from build123d import *

# Parameters (mm, degrees)
SKETCH2_W                                           = 150
SKETCH2_H                                           = 30
BOSS_EXTRUDE1_DEPTH                                 = 20
SKETCH3_R                                           = 13.75
CUT_EXTRUDE1_DEPTH                                  = 13
LPATTERN1_COUNT                                     = 5
LPATTERN1_PITCH                                     = 30
CBORE_FOR_M4_HEX_SOCKET_HEAD_CAP_SCREW1_D           = 4.5
CBORE_FOR_M4_HEX_SOCKET_HEAD_CAP_SCREW1_CBORE_D     = 8
CBORE_FOR_M4_HEX_SOCKET_HEAD_CAP_SCREW1_CBORE_DEPTH = 4.4
LPATTERN2_COUNT                                     = 2
LPATTERN2_PITCH                                     = 120
SKETCH7_W                                           = 181.12901383
SKETCH7_H                                           = 4
CUT_EXTRUDE3_DEPTH                                  = 13
SKETCH8_W                                           = 4
SKETCH8_H                                           = 50
CUT_EXTRUDE4_DEPTH                                  = 13
LPATTERN3_COUNT                                     = 5
LPATTERN3_PITCH                                     = 30


with BuildPart() as part:
    # Sketch2 → Boss-Extrude1 (new body)
    with BuildSketch(Plane(origin=(0, 0, 0), x_dir=(1, 0, 0), z_dir=(0, 1, 0))):
        Rectangle(SKETCH2_W, SKETCH2_H)
    extrude(amount=BOSS_EXTRUDE1_DEPTH)

    # Sketch3 → Cut-Extrude1 (cut)
    with BuildSketch(Plane(origin=(0, 20, 0), x_dir=(1, 0, 0), z_dir=(0, 1, 0))):
        with Locations(Location((-60, 0, 0), (0, 0, 270))):
            Circle(SKETCH3_R)
    cut_extrude1 = extrude(amount=-CUT_EXTRUDE1_DEPTH, mode=Mode.SUBTRACT)

    # LPattern1: Cut-Extrude1 ×5
    with Locations(*[(i * LPATTERN1_PITCH, 0, 0) for i in range(1, LPATTERN1_COUNT)]):
        add(cut_extrude1, mode=Mode.SUBTRACT)

    # CBORE for M4 Hex Socket Head Cap Screw1 (through all)
    with Locations(Plane(origin=(0, 7, 0), x_dir=(-1, 0, 0), z_dir=(0, 1, 0))):
        with Locations((60, 0)):
            cbore_for_m4_hex_socket_head_cap_screw1 = CounterBoreHole(CBORE_FOR_M4_HEX_SOCKET_HEAD_CAP_SCREW1_D / 2, CBORE_FOR_M4_HEX_SOCKET_HEAD_CAP_SCREW1_CBORE_D / 2, CBORE_FOR_M4_HEX_SOCKET_HEAD_CAP_SCREW1_CBORE_DEPTH)

    # LPattern2: CBORE for M4 Hex Socket Head Cap Screw1 ×2
    with Locations(*[(i * LPATTERN2_PITCH, 0, 0) for i in range(1, LPATTERN2_COUNT)]):
        add(cbore_for_m4_hex_socket_head_cap_screw1, mode=Mode.SUBTRACT)

    # Sketch7 → Cut-Extrude3 (cut)
    with BuildSketch(Plane(origin=(0, 20, 0), x_dir=(1, 0, 0), z_dir=(0, 1, 0))):
        Rectangle(SKETCH7_W, SKETCH7_H)
    extrude(amount=-CUT_EXTRUDE3_DEPTH, mode=Mode.SUBTRACT)

    # Sketch8 → Cut-Extrude4 (cut)
    with BuildSketch(Plane(origin=(0, 20, 0), x_dir=(-1, 0, 0), z_dir=(0, 1, 0))):
        with Locations((60, -1.298701607)):
            Rectangle(SKETCH8_W, SKETCH8_H)
    cut_extrude4 = extrude(amount=-CUT_EXTRUDE4_DEPTH, mode=Mode.SUBTRACT)

    # LPattern3: Cut-Extrude4 ×5
    with Locations(*[(i * LPATTERN3_PITCH, 0, 0) for i in range(1, LPATTERN3_COUNT)]):
        add(cut_extrude4, mode=Mode.SUBTRACT)


solid = part.part
The listing builds one solid part. Answer for the finished solid, in the listing's coordinates (mm). A direction names the side the tool comes from. Coordinates: 2 decimals unless noted, no trailing zeros. Write each loop counter-clockwise with the first axis right and the second up, starting at its lowest first coordinate (ties: lowest second). Pieces come first, ordered by that corner, then holes. Notation, with made-up numbers: (11, 66) -> (45, 66) arc R17 cw to (45, 73) -> close; hole circle Ø3 at (-21, -21.75). An arc over 180 degrees is marked (long way). One line per question, with ' | ' between items.
1. Section A-A (z = 0) is taken. Determine the outline of the cut face in (x, y).
Verdict:
outline: (-75, 0) -> (-62.25, 0) -> (-62.25, 2.6) -> (-64, 2.6) -> (-64, 7) -> (-75, 7) -> close; (-57.75, 0) -> (57.75, 0) -> (57.75, 2.6) -> (56, 2.6) -> (56, 7) -> (-56, 7) -> (-56, 2.6) -> (-57.75, 2.6) -> close; (62.25, 0) -> (75, 0) -> (75, 7) -> (64, 7) -> (64, 2.6) -> (62.25, 2.6) -> close
2. Section B-B (x = 60) is taken. Determine the outline of the cut face in (y, z).
Verdict:
outline: (0, -15) -> (7, -15) -> (7, -4) -> (2.6, -4) -> (2.6, -2.25) -> (0, -2.25) -> close; (0, 2.25) -> (2.6, 2.25) -> (2.6, 4) -> (7, 4) -> (7, 15) -> (0, 15) -> close
3. Given pin 1 Ø5 at (x, z) = (60, 0) entering from +Y; pin 2 Ø8 at (x, z) = (29.5, -6) entering from +Y, each flat-ended and moving along its own axis, determine where each tip first touches the part or whether it passes through.
Verdict:
pin 1: stops at y = 2.6 | pin 2: stops at y = 7
4. Section C-C (z = 5.5) is taken. Determine the outline of the cut face in (x, y), and give its area (3 significant figures).
Verdict:
outline: (-75, 0) -> (75, 0) -> (75, 20) -> (72.6, 20) -> (72.6, 7) -> (47.4, 7) -> (47.4, 20) -> (42.6, 20) -> (42.6, 7) -> (17.4, 7) -> (17.4, 20) -> (12.6, 20) -> (12.6, 7) -> (-12.6, 7) -> (-12.6, 20) -> (-17.4, 20) -> (-17.4, 7) -> (-42.6, 7) -> (-42.6, 20) -> (-47.4, 20) -> (-47.4, 7) -> (-72.6, 7) -> (-72.6, 20) -> (-75, 20) -> close | area: 1,360 mm^2
5. Section D-D (y = 9) is taken. State how many separate pieces and enclosed holes the cut face has, and give its area (3 significant figures).
Verdict:
separate pieces: 12 | enclosed holes: 0 | area: 1,430 mm^2
6. Straight lines are drawn through the part: line 1 (Z direction, x = 60, y = 0.5); line 2 (X direction, y = 13.5, z = 10); line 3 (X direction, y = 10.25, z = -2.5). For each, find the intervals that lie inside material, in ascending order.
Verdict:
line 1: z = -15 to -2.25, 2.25 to 15 | line 2: x = -75 to -69.44, -50.56 to -39.44, -20.56 to -9.44, 9.44 to 20.56, 39.44 to 50.56, 69.44 to 75 | line 3: x = -75 to -73.52, -46.48 to -43.52, -16.48 to -13.52, 13.52 to 16.48, 43.52 to 46.48, 73.52 to 75
7. For a pull along X with two mould halves and no side action, classify faces 1 (the cylindrical face through (-39.635, 13.591, -9.809)), 2 (the cylindrical face through (57.752, 1.282, 0.099)), 3 (the flat face through (45, 20, -11)) as released by +X, released by -X, zero draft, split by the parting line, or undercut.
Verdict:
face 1: undercut | face 2: undercut | face 3: zero draft
8. Which of the six approach directions +Z, -Z, +X, -X, +Y, -Y give full straight-line access (tool end or side, diameter ignored) to faces 4 (the cylindrical face through (-20.191, 13.591, -9.635)), 5 (the flat face through (-15, 14, 2)), 6 (the flat face through (-71, 20, 11))?
Verdict:
face 4: +Y | face 5: +X, -X, +Y | face 6: +Z, -Z, +X, -X, +Y
